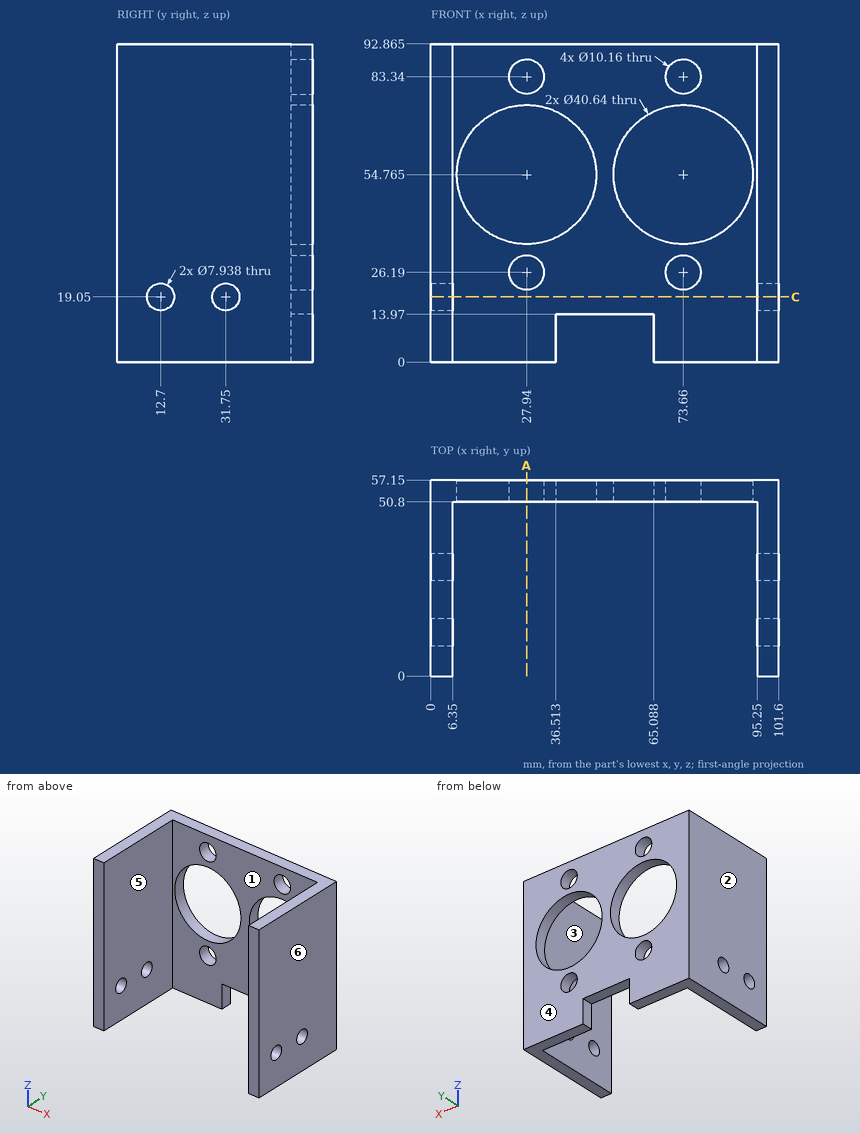
The figure shows three views and two pictorial views of one solid part (mm, origin at its lowest corner). Answer the questions. A direction names the side the tool comes from. Round coordinates to 2 decimals unless told otherwise and drop trailing zeros. Loops run counter-clockwise (first coordinate to the right, second up) from the corner with the lowest first, then second, coordinate; pieces in that order, holes last. Notation, with made-up numbers: M 41.25,9 L 71.25,9 A14 cw 71.25,20 Z; hole C 79.25,-40 d6. An arc over 180 degrees is marked long. Return JSON: item names as keys, results as strings.
Q1. Find the intervals of material crossed by line 1 along X through (y, z) = (55, 83); line 2 along Y through (x, z) = (99.5, 19.05); line 3 along Z through (x, y) = (73.66, 53.25) (1 decimal), in increasing order. Write a range as from..to.
Results list:
{"line 1": "x = 0..22.87, 33.01..68.59, 78.73..101.6", "line 2": "y = 0..8.73, 16.67..27.78, 35.72..57.15", "line 3": "z = 0..21.1, 31.3..34.4, 75.1..78.3, 88.4..92.9"}
Q2. Which of the six approach directions +Z, -Z, +X, -X, +Y, -Y give full straight-line access (tool end or side, diameter ignored) to the marked faces 5 and 6?
Results list:
{"face 5": "+Z, -Z, -Y", "face 6": "+Z, -Z, +X, +Y, -Y"}
Q3. This flat-tipped pin is pushed along its axis until it touches: pin 1 Ø11.5 at (x, z) = (27.94, 83.34) entering from -Y. Where does it stop, or does it pass through?
Results list:
{"pin 1": "stops at y = 50.8"}
Q4. Find section A-A, the plane x = 27.94. State how many separate pieces and enclosed holes the cut face has.
Results list:
{"separate pieces": "4", "enclosed holes": "0"}
Q5. The mould has two halves that part along X. Classify the marked faces 1, 2, 3 and 4: released by +X, released by -X, zero draft, split by the parting line, or undercut.
Results list:
{"face 1": "undercut", "face 2": "released by -X", "face 3": "undercut", "face 4": "zero draft"}
Q6. Find section C-C, the plane z = 19.05. Determine the outline of the cut face in (x, y), plus the area to 3 significant figures.
Results list:
{"outline": "M 0,0 L 6.35,0 L 6.35,8.73 L 0,8.73 Z; M 0,16.67 L 6.35,16.67 L 6.35,27.78 L 0,27.78 Z; M 0,35.72 L 6.35,35.72 L 6.35,50.8 L 95.25,50.8 L 95.25,35.72 L 101.6,35.72 L 101.6,57.15 L 0,57.15 Z; M 95.25,0 L 101.6,0 L 101.6,8.73 L 95.25,8.73 Z; M 95.25,16.67 L 101.6,16.67 L 101.6,27.78 L 95.25,27.78 Z", "area": "1,090 mm2"}
